Here's how the part is built. I have some questions about the finished solid (model axes, mm). A direction names the side the tool comes from. Round coordinates to 2 decimals unless told otherwise and drop trailing zeros. Loops run counter-clockwise (first coordinate to the right, second up) from the corner with the lowest first, then second, coordinate; pieces in that order, holes last. Notation, with made-up numbers: M 85,13.5 L 127,13.5 A18 cw 127,21.5 Z; hole C 14,43 d7. An arc over 180 degrees is marked long. Put each result on its own line as item: value. Start each with the question number.
```python
from build123d import *

# Parameters (mm, degrees)
F1_DEPTH = 19.05
F2_W     = 70.8835957375
F2_H     = 27.94
F3_DEPTH = 3.175
F4_R     = 12.6886346665
F5_DEPTH = 14.732


# Not quite as in the source:
# - a fillet or chamfer that OpenCascade refuses, or shapes differently, is made with other operations: its cross-section is extruded or revolved along the edge and cut away or added


with BuildPart() as f1:
    # F0 (on Top) → F1 (new body)
    with BuildSketch(Plane.XY):
        Polygon((-16.5059205686, -50.8), (16.5059205686, -50.8), (43.2130610643, -31.3961266285), (53.4142809913, 0), (43.2130610643, 31.3961266285), (16.5059205686, 50.8), (-16.5059205686, 50.8), (-43.2130610643, 31.3961266285), (-53.4142809913, 0), (-43.2130610643, -31.3961266285), align=None)
    extrude(amount=F1_DEPTH)

    # F2 (on face) → F3 (join)
    with BuildSketch(Plane(origin=(0, 0, 0), x_dir=(1, 0, 0), z_dir=(0, 0, -1))):
        Rectangle(F2_W, F2_H)
    extrude(amount=F3_DEPTH)

    # F4 (on face) → F5 (join)
    with BuildSketch(Plane(origin=(0, 0, -3.175), x_dir=(1, 0, 0), z_dir=(0, 0, -1))):
        Circle(F4_R)
    extrude(amount=F5_DEPTH)

    # F6: chamfer of 12.6873 x 15.1201353553 on 1 edges, made by hand


with BuildPart() as f6_tool2:
    # F6_s3 → F6_t4 (revolve)
    with BuildSketch(Plane.XZ):
        Polygon((12.6886346665, -2.7868646447), (0.0013346665, -17.907), (12.6886346665, -17.907), align=None)
    revolve(axis=Axis((0, 0, -17.907), (0, 0, -1)))

    split(bisect_by=Plane.XY.offset(-3.175), keep=Keep.BOTTOM)


with BuildPart() as f1_1:
    add(f1.part)

    # F6_t1: cut F6_tool2
    add(f6_tool2.part, mode=Mode.SUBTRACT)


solid = f1_1.part
```
1) Suppose I cut it at A-A (z = 9.5). Write out the boundary of the cut face in (x, y).
2) Suppose I cut it at D-D (x = -31.5). Write out the boundary of the cut face in (y, z) (3 decimals), plus the area to 3 significant figures.
3) Suppose I cut it at B-B (x = 25). Write out the boundary of the cut face in (y, z) (3 decimals), plus the area to 3 significant figures.
4) If I drill on probe 1 along Z at (x, y) = (-20, -21); probe 2 along X at (y, z) = (4, -6); probe 3 along X at (y, z) = (22, 1.5), over which ranges is the centre line in solid material (lowest first)? Write a range as from..to.
5) On a 3-axis mill with a long thin cutter (end or side, diameter ignored), from which of +Z, -Z, +X, -X, +Y, -Y can I reach the whole of each face in a straight line? I mean faces 1 (the face through (0, -13.97, -2)), 2 (the face through (0, 13.97, -2)), 3 (the face through (-35.442, 0, -2)), 4 (the face through (35.442, 0, -2)). Say none if no direction works.
6) Suppose I cut it at C-C (y = -34.5). Write out the boundary of the cut face in (x, z).
7) I'm going to push flat-ended pins straight in: P1, Ø3.5, axis at y = 5.5, z = -2, coming from the -X side; P2, Ø1.6, axis at y = 6.5, z = -1, coming from the +X side; P3, Ø10, axis at y = -17, z = 2.5, coming from the -X side. Where does each tip first touch, or does it pass through?
Results are:
1. outline: M -53.41,0 L -43.21,-31.4 L -16.51,-50.8 L 16.51,-50.8 L 43.21,-31.4 L 53.41,0 L 43.21,31.4 L 16.51,50.8 L -16.51,50.8 L -43.21,31.4 Z
2. outline: M -39.906,0 L -13.97,0 L -13.97,-3.175 L 13.97,-3.175 L 13.97,0 L 39.906,0 L 39.906,19.05 L -39.906,19.05 Z
2. area: 1,610 mm²
3. outline: M -44.629,0 L -13.97,0 L -13.97,-3.175 L 13.97,-3.175 L 13.97,0 L 44.629,0 L 44.629,19.05 L -44.629,19.05 Z
3. area: 1,790 mm²
4. probe 1: 0..19.05
4. probe 2: -9.16..9.16
4. probe 3: -46.27..46.27
5. face 1: -Z, +X, -X, -Y
5. face 2: -Z, +X, -X, +Y
5. face 3: -Z, -X, +Y, -Y
5. face 4: -Z, +X, +Y, -Y
6. outline: M -38.94,0 L 38.94,0 L 38.94,19.05 L -38.94,19.05 Z
7. P1: x = -35.44
7. P2: x = 35.44
7. P3: x = -49.52
